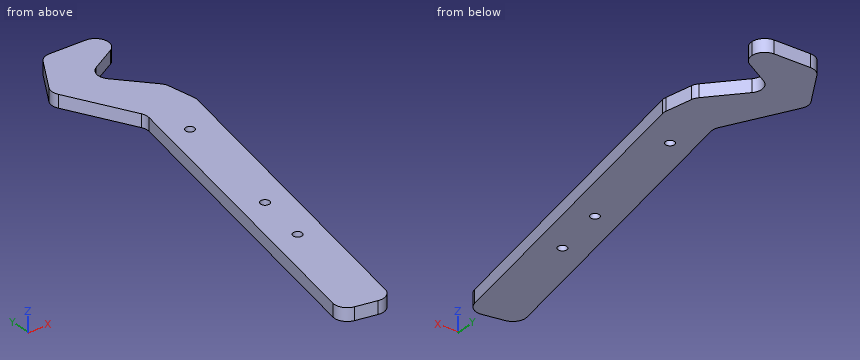
```python
from build123d import *

# Parameters (mm, degrees)
SKETCH1_R           = 1.7
BOSS_EXTRUDE1_DEPTH = 5


with BuildPart() as part:
    # Sketch1 → Boss-Extrude1 (new body)
    with BuildSketch(Plane.XY):
        with BuildLine():
            Line((-6.070464182, 24.812225303), (-19.958071354, 25.288330369))
            ThreePointArc((-19.958071354, 25.288330369), (-22.490276705, 24.698780913), (-24.384131469, 22.917504226))
            Line((-24.384131469, 22.917504226), (-32.767669467, 9.335402505))
            ThreePointArc((-32.767669467, 9.335402505), (-33.509344938, 6.898271001), (-32.954010567, 4.412049729))
            Line((-32.954010567, 4.412049729), (-19.944783446, -20.739122704))
            ThreePointArc((-19.944783446, -20.739122704), (-19.435661169, -22.332379304), (-19.480501521, -24.004402458))
            Line((-19.480501521, -24.004402458), (-43.771872125, -147.080680186))
            ThreePointArc((-43.771872125, -147.080680186), (-43.019718624, -150.832869688), (-39.834667143, -152.954215487))
            Line((-39.834667143, -152.954215487), (-31.766323039, -154.546651824))
            ThreePointArc((-31.766323039, -154.546651824), (-28.014133538, -153.794498323), (-25.892787738, -150.609446842))
            Line((-25.892787738, -150.609446842), (-1.06250464, -24.802679145))
            ThreePointArc((-1.06250464, -24.802679145), (-0.968074634, -23.879218397), (-1.045977095, -22.954216783))
            Line((-1.045977095, -22.954216783), (-2.879406447, -12.703188307))
            ThreePointArc((-2.879406447, -12.703188307), (-3.295898049, -11.415233674), (-4.042598503, -10.286193895))
            Line((-4.042598503, -10.286193895), (-15.024159675, 2.232097065))
            ThreePointArc((-15.024159675, 2.232097065), (-16.188614474, 6.402596208), (-13.660892318, 9.918224001))
            Line((-13.660892318, 9.918224001), (-3.844891775, 15.275823833))
            ThreePointArc((-3.844891775, 15.275823833), (-1.928275453, 17.133614871), (-1.240561171, 19.712733856))
            Line((-1.240561171, 19.712733856), (-1.242008304, 19.86323568))
            ThreePointArc((-1.242008304, 19.86323568), (-2.662930088, 23.306844453), (-6.070464182, 24.812225303))
        make_face()
        with Locations((-13.865353247, -37.357391651)):
            Circle(SKETCH1_R, mode=Mode.SUBTRACT)
        with Locations((-26.748462507, -107.729710298)):
            Circle(SKETCH1_R, mode=Mode.SUBTRACT)
        with Locations((-22.825562759, -86.412593899)):
            Circle(SKETCH1_R, mode=Mode.SUBTRACT)
    extrude(amount=BOSS_EXTRUDE1_DEPTH)


solid = part.part
```
Geometry check sheet. Reference: the model listing, model coordinates, mm. Give positions to 0.01 mm unless a question says otherwise; leave off trailing zeros. Write each loop counter-clockwise with the first axis right and the second up, starting at its lowest first coordinate (ties: lowest second). Pieces come first, ordered by that corner, then holes.
1) Material ranges on L1, parallel to X at y = -23.5, z = 0.45; L2, parallel to X at y = -66.5, z = 4.85, recorded low to high.
2) Section check B-B, the plane z = 1.3. Record the boundary of the cut face in (x, y).
3) Section check D-D, the plane y = -18. Record the boundary of the cut face in (x, z).
4) Section check A-A, the plane x = -8. Record the boundary of the cut face in (y, z) (3 decimals).
5) Gauge pin test, flat ends, axial feed: pin 1 (3 mm diameter, centred on y = -84.5, z = 1, fed in from +X); pin 2 (1.5 mm diameter, centred on x = -32, z = 1.5, fed in from -Y). Record the tip position at first contact, or that the pin passes through.
6) Section check C-C, the plane y = -134. Record the boundary of the cut face in (x, z), and give its area (3 significant figures).
Computed:
1. L1: x = -19.41 to -0.98
1. L2: x = -27.87 to -9.29
2. outline: (-43.77, -147.08) arc R5 ccw to (-39.83, -152.95) - (-31.77, -154.55) arc R5 ccw to (-25.89, -150.61) - (-1.06, -24.8) arc R5 ccw to (-1.05, -22.95) - (-2.88, -12.7) arc R5 ccw to (-4.04, -10.29) - (-15.02, 2.23) arc R5 cw to (-13.66, 9.92) - (-3.84, 15.28) arc R5 ccw to (-1.24, 19.71) - (-1.24, 19.86) arc R5 ccw to (-6.07, 24.81) - (-19.96, 25.29) arc R5 ccw to (-24.38, 22.92) - (-32.77, 9.34) arc R5 ccw to (-32.95, 4.41) - (-19.94, -20.74) arc R5 cw to (-19.48, -24) - close; hole circle Ø3.4 at (-26.75, -107.73); hole circle Ø3.4 at (-22.83, -86.41); hole circle Ø3.4 at (-13.87, -37.36)
3. outline: (-21.36, 0) - (-1.93, 0) - (-1.93, 5) - (-21.36, 5) - close
4. outline: (-59.953, 0) - (-5.775, 0) - (-5.775, 5) - (-59.953, 5) - close; (13.008, 0) - (24.878, 0) - (24.878, 5) - (13.008, 5) - close
5. pin 1: stops at x = -12.55
5. pin 2: stops at y = -154.62
6. outline: (-41.19, 0) - (-22.61, 0) - (-22.61, 5) - (-41.19, 5) - close
6. area: 92.9 mm2
